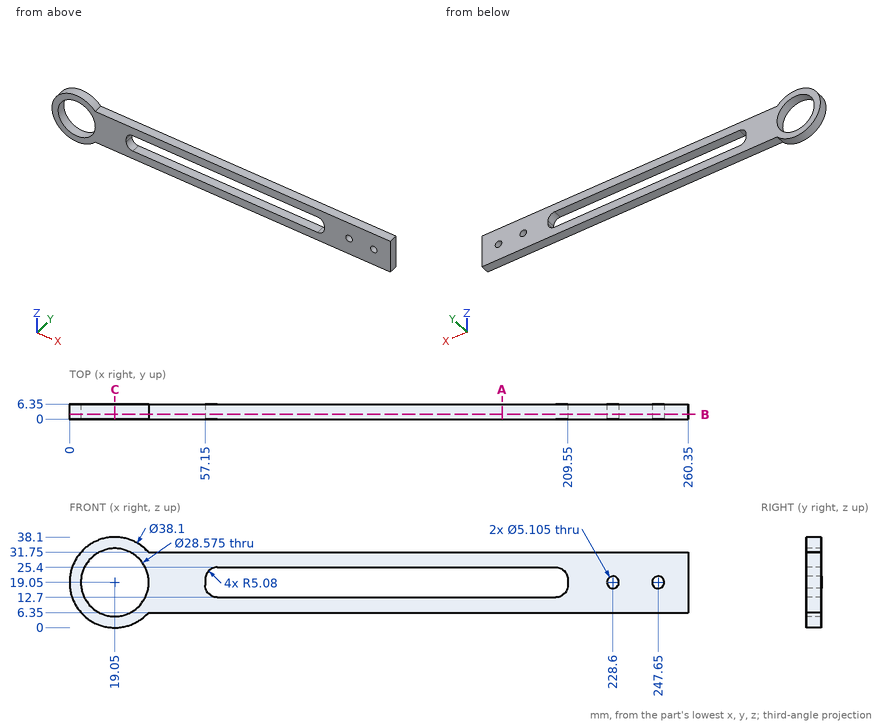
Can you work these out from the drawing? Everything is in mm from the part's minimum corner. Coordinates: 2 decimals unless noted, no trailing zeros. Loops run counter-clockwise (first coordinate to the right, second up) from the corner with the lowest first, then second, coordinate; pieces in that order, holes last. Notation, with made-up numbers: M -40,66 L 11,66 A34 ccw 11,100 Z; hole C 60.5,-24 d8. An arc over 180 degrees is marked long. Put each result on its own line as item: value. Start each with the question number.
(1) Suppose I cut it at B-B on y = 2. Count the separate pieces of the cut face and the enclosed holes in it, then the cut area to 3 significant figures.
(2) Will these pins go through, and if not, where does the flat tip stop? P1, Ø0.8, axis at y = 3, z = 19.5, coming from the -X side; P2, Ø3, axis at x = 172, y = 1, coming from the -Z side; P3, Ø1.9, axis at x = 111.5, y = 2, coming from the +Z side; P4, Ø4.5, axis at x = 228.6, z = 19.05, coming from the +Y side.
(3) Suppose I cut it at C-C on x = 19.05. Please give me the cut outline in (y, z).
(4) I need wall thicknesses on line 1 (X direction, y = 3.5, z = 19.05); line 2 (Z direction, x = 73.5, y = 1.25); line 3 (Z direction, x = 247.65, y = 3.25). Which ranges of each line are inside material? Lowest first, please. Write a range as from..to.
(5) Suppose I cut it at A-A on x = 182. Please give me the cut outline in (y, z).
Solutions:
1. separate pieces: 1
1. enclosed holes: 4
1. area: 4,230 mm2
2. P1: stops at x = 0
2. P2: stops at z = 6.35
2. P3: stops at z = 31.75
2. P4: passes through
3. outline: M 0,0 L 6.35,0 L 6.35,4.76 L 0,4.76 Z; M 0,33.34 L 6.35,33.34 L 6.35,38.1 L 0,38.1 Z
4. line 1: x = 0..4.76, 33.34..57.15, 209.55..226.05, 231.15..245.1, 250.2..260.35
4. line 2: z = 6.35..12.7, 25.4..31.75
4. line 3: z = 6.35..16.5, 21.6..31.75
5. outline: M 0,6.35 L 6.35,6.35 L 6.35,12.7 L 0,12.7 Z; M 0,25.4 L 6.35,25.4 L 6.35,31.75 L 0,31.75 Z
